Work out the finished part from the listing and answer in its coordinate system (mm). Give positions to 0.01 mm unless a question says otherwise; leave off trailing zeros. Write each loop counter-clockwise with the first axis right and the second up, starting at its lowest first coordinate (ties: lowest second). Pieces come first, ordered by that corner, then holes. Notation, with made-up numbers: (-27, 69) -> (32, 69) arc R11 cw to (32, 88) -> close; hole circle Ø1 at (-2, -15.5). An arc over 180 degrees is marked (long way). Write item = value, one per line. Start each with the question number.
from build123d import *

# Parameters (mm, degrees)
SKETCH1_R           = 8
BOSS_EXTRUDE1_DEPTH = 3


with BuildPart() as part:
    # Sketch1 → Boss-Extrude1 (new body)
    with BuildSketch(Plane.XY):
        Polygon((-10.5, -24.5), (0, -24.5), (10.5, -24.5), (10.5, -27.5), (31.5, -27.5), (31.5, -24.5), (52.5, -24.5), (52.5, -27.5), (73.5, -27.5), (73.5, -24.5), (95, -24.5), (95, -10), (98, -10), (98, 10), (95, 10), (95, 27.5), (-95, 27.5), (-95, 10), (-98, 10), (-98, -10), (-95, -10), (-95, -24.5), (-73.5, -24.5), (-73.5, -27.5), (-52.5, -27.5), (-52.5, -24.5), (-31.5, -24.5), (-31.5, -27.5), (-10.5, -27.5), align=None)
        with Locations((-34.4, 11)):
            Circle(SKETCH1_R, mode=Mode.SUBTRACT)
        with Locations((34.4, 11)):
            Circle(SKETCH1_R, mode=Mode.SUBTRACT)
    extrude(amount=BOSS_EXTRUDE1_DEPTH)


solid = part.part
(1) A cutting plane is placed at B-B, the plane z = 0.75. State how many separate pieces and enclosed holes the cut face has, then the cut area to 3 significant figures.
(2) Determine the mould class of faces 1 (the cylindrical face through (-36.13, 3.19, 1.48)), 2 (the flat face through (-1, 0, 3)) for opening direction X: pulls with the +X half, pulls with the -X half, needs draft (parallel to the pull), parting line crosses it, or undercut.
(3) A cutting plane is placed at C-C, the plane y = 15.5. Write down the section's boundary in (x, z).
(4) A cutting plane is placed at A-A, the plane x = -34.4. Write down the section's boundary in (y, z), then the cut area to 3 significant figures.
(5) A cutting plane is placed at D-D, the plane y = 23.5. Write down the section's boundary in (x, z), then the cut area to 3 significant figures.
(6) Find the intervals of material crossed by line 1 along Y through (x, z) = (34.4, 1.1); line 2 along X through (y, z) = (25.5, 2.1); line 3 along X through (y, z) = (6, 1.45) (3 decimals), in increasing order.
(7) Each of these flat-tipped pins is pushed along its axis until it touches: pin 1 (0.9 mm diameter, centred on x = 45, z = 1, fed in from -Y); pin 2 (1.5 mm diameter, centred on x = 96.5, z = 1, fed in from -Y); pin 3 (1 mm diameter, centred on y = -19.5, z = 2.5, fed in from -X). Where does it stop, or does it pass through?
Results list:
q1.separate_pieces = 1
q1.enclosed_holes = 2
q1.area = 9,850 mm²
q2.face_1 = undercut
q2.face_2 = needs draft
q3.outline = (-95, 0) -> (-41.01, 0) -> (-41.01, 3) -> (-95, 3) -> close; (-27.79, 0) -> (27.79, 0) -> (27.79, 3) -> (-27.79, 3) -> close; (41.01, 0) -> (95, 0) -> (95, 3) -> (41.01, 3) -> close
q4.outline = (-24.5, 0) -> (3, 0) -> (3, 3) -> (-24.5, 3) -> close; (19, 0) -> (27.5, 0) -> (27.5, 3) -> (19, 3) -> close
q4.area = 108 mm²
q5.outline = (-95, 0) -> (95, 0) -> (95, 3) -> (-95, 3) -> close
q5.area = 570 mm²
q6.line_1 = -24.5 to 3, 19 to 27.5
q6.line_2 = -95 to 95
q6.line_3 = -98 to -40.645, -28.155 to 28.155, 40.645 to 98
q7.pin_1 = -24.5
q7.pin_2 = -10
q7.pin_3 = -95
